Could you check a few things on this drawing? It's one solid part, dimensions in mm from its lowest x, y, z. A direction names the side the tool comes from. Give positions to 0.01 mm unless a question says otherwise; leave off trailing zeros. Loops run counter-clockwise (first coordinate to the right, second up) from the corner with the lowest first, then second, coordinate; pieces in that order, holes last. Notation, with made-up numbers: M -29.5,57.5 L -16.5,57.5 A27 cw -16.5,90.5 Z; hole C 72,60 d8. An arc over 180 degrees is marked long. Answer as a JSON object with one key per item and string values.
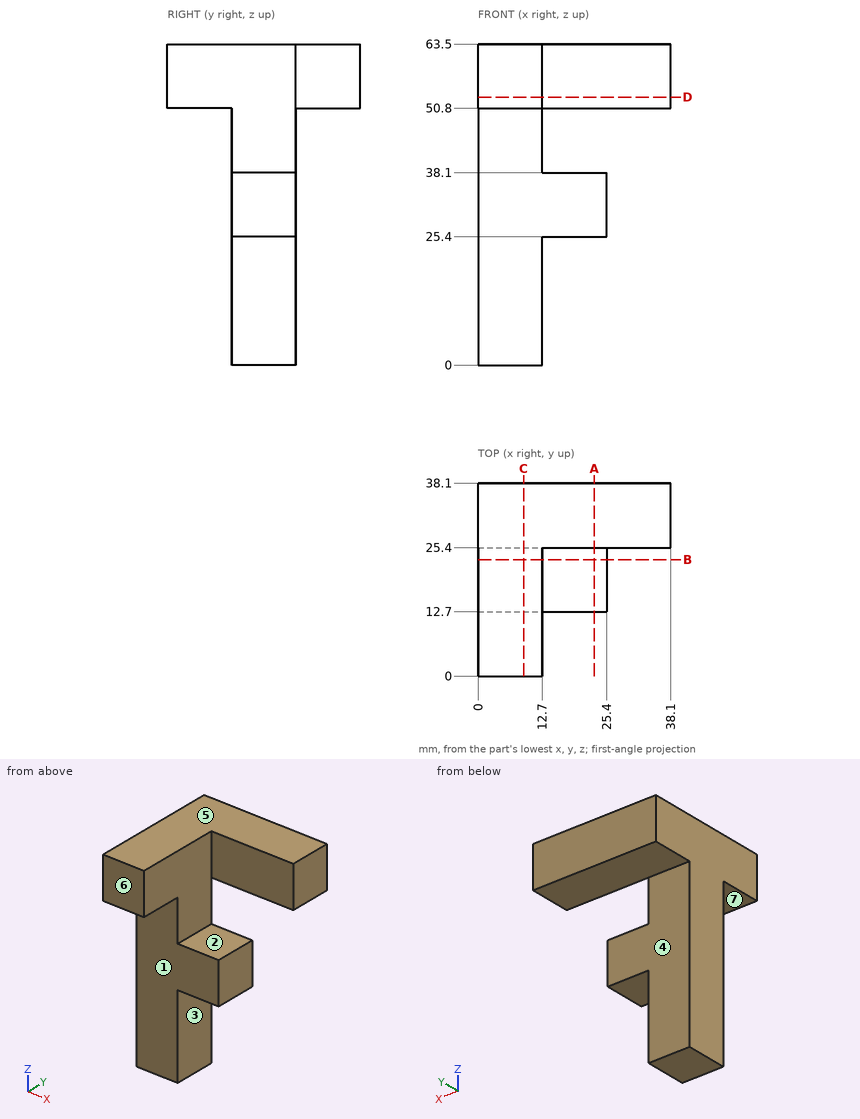
1) For the marked faces 1, 2, 3 and 4, which set-ups out of +Z, -Z, +X, -X, +Y, -Y let a thin tool reach every point of the face, with its end or its side?
Answer list:
{"face 1": "-Z, +X, -X, -Y", "face 2": "+Z, +X, +Y, -Y", "face 3": "-Z, +X, +Y, -Y", "face 4": "-Z, +X, -X, +Y"}
2) Will these pins go through, and if not, where does the flat tip stop? pin 1 Ø6.5 at (x, y) = (13, 35) entering from -Z; pin 2 Ø8 at (x, y) = (23, 11.5) entering from +Z; pin 3 Ø6 at (y, z) = (13.5, 6.5) entering from +X.
Answer list:
{"pin 1": "z = 50.8", "pin 2": "z = 38.1", "pin 3": "x = 12.7"}
3) If we mould it in two halves opening along Z, with no side actions, what happens to the marked faces 5, 6 and 7? For each: +Z half, -Z half, draft (parallel to the pull), parting line (faces both ways), or undercut.
Answer list:
{"face 5": "+Z half", "face 6": "draft", "face 7": "-Z half"}
4) Suppose I cut it at A-A, the plane x = 23. Write out the boundary of the cut face in (y, z), and give its area (3 significant figures).
Answer list:
{"outline": "M 12.7,25.4 L 25.4,25.4 L 25.4,38.1 L 12.7,38.1 Z; M 25.4,50.8 L 38.1,50.8 L 38.1,63.5 L 25.4,63.5 Z", "area": "323 mm^2"}
5) Please list where these lines run through material, in increasing order: line 1 along X through (y, z) = (7.5, 55); line 2 along Y through (x, z) = (18, 32.5); line 3 along Z through (x, y) = (22, 28). Write a range as from..to.
Answer list:
{"line 1": "0..12.7", "line 2": "12.7..25.4", "line 3": "50.8..63.5"}
6) Suppose I cut it at D-D, the plane z = 53. Write out the boundary of the cut face in (x, y), and give its area (3 significant figures).
Answer list:
{"outline": "M 0,0 L 12.7,0 L 12.7,25.4 L 38.1,25.4 L 38.1,38.1 L 0,38.1 Z", "area": "806 mm^2"}
7) Suppose I cut it at C-C, the plane x = 9. Write out the boundary of the cut face in (y, z).
Answer list:
{"outline": "M 0,50.8 L 12.7,50.8 L 12.7,0 L 25.4,0 L 25.4,50.8 L 38.1,50.8 L 38.1,63.5 L 0,63.5 Z"}
8) Suppose I cut it at B-B, the plane y = 23. Write out the boundary of the cut face in (x, z).
Answer list:
{"outline": "M 0,0 L 12.7,0 L 12.7,25.4 L 25.4,25.4 L 25.4,38.1 L 12.7,38.1 L 12.7,63.5 L 0,63.5 Z"}
